```python
from build123d import *

# Parameters (mm, degrees)
F0_W     = 15
F0_H     = 90
F0_R     = 1.5
F1_DEPTH = 3
F2_W     = 15
F2_H     = 3
F3_DEPTH = 17
F4_R     = 2.5
F5_DEPTH = 53.001


with BuildPart() as f1:
    # F0 (on Front) → F1 (new body)
    with BuildSketch(Plane.XZ):
        Rectangle(F0_W, F0_H)
        with Locations((0, -41)):
            Circle(F0_R, mode=Mode.SUBTRACT)
        with Locations((0, 41)):
            Circle(F0_R, mode=Mode.SUBTRACT)
    extrude(amount=F1_DEPTH)

    # F2 (on face) → F3 (join)
    with BuildSketch(Plane.XZ.offset(3)):
        with Locations((0, 6.5)):
            Rectangle(F2_W, F2_H)
    extrude(amount=F3_DEPTH)

    # F4 (on face) → F5 (cut, through all)
    with BuildSketch(Plane.XY.offset(8)):
        with Locations((0, -11.5)):
            Circle(F4_R)
    extrude(amount=-F5_DEPTH, mode=Mode.SUBTRACT)


solid = f1.part
```
The model under review builds one solid part; all positions refer to its coordinate system, in mm. A direction names the side the tool comes from. Coordinates: 2 decimals unless noted, no trailing zeros. Write each loop counter-clockwise with the first axis right and the second up, starting at its lowest first coordinate (ties: lowest second). Pieces come first, ordered by that corner, then holes.
1) The part is to be moulded in two halves that separate along X. For faces 4 (the face through (0, -3, -20)), 5 (the face through (7.5, -2.5, -0.2)), 6 (the face through (-0.325, -1.479, 39.536)), say which applies: pulls with the +X half, pulls with the -X half, needs draft (parallel to the pull), parting line crosses it, or undercut.
2) We need section C-C on x = 0. State the section outline as (y, z) points.
3) We need section A-A on z = 41. State the section outline as (x, y) points.
4) We need section D-D on x = 6. State the section outline as (y, z) points, then the cut area to 3 significant figures.
5) Clearance check with flat-ended pins moving along their axes: pin 1 Ø12 at (y, z) = (-7, 15.5) entering from +X; pin 2 Ø6 at (x, y) = (0, -11.5) entering from -Z; pin 3 Ø7.5 at (x, z) = (-3.5, 20.5) entering from -Y; pin 4 Ø2 at (x, y) = (0.5, -15.5) entering from +Z. State where each tip first meets the part, or that it passes through.
6) To check wall thickness, follow probe 1 along Z at (x, y) = (0, -2.4); probe 2 along Z at (x, y) = (-3, -4); probe 3 along Y at (x, z) = (5.75, -26). State the ranges of each line that lie inside material, in increasing order.
7) We need section B-B on y = -13. State the section outline as (x, z) points.
8) Machinability: for faces 1 (the face through (-2, -9, 5)), 2 (the face through (-7.5, -2.5, -0.2)), 3 (the face through (-2, -9, 8)), which of the approach directions +Z, -Z, +X, -X, +Y, -Y give a long, thin tool a straight path to every point of the face, cutting with its end or side? Answer none if there is none.
Answer list:
1. face 4: needs draft
1. face 5: pulls with the +X half
1. face 6: undercut
2. outline: (-20, 5) - (-14, 5) - (-14, 8) - (-20, 8) - close; (-9, 5) - (-3, 5) - (-3, -39.5) - (0, -39.5) - (0, 39.5) - (-3, 39.5) - (-3, 8) - (-9, 8) - close; (-3, -45) - (0, -45) - (0, -42.5) - (-3, -42.5) - close; (-3, 42.5) - (0, 42.5) - (0, 45) - (-3, 45) - close
3. outline: (-7.5, -3) - (-1.5, -3) - (-1.5, 0) - (-7.5, 0) - close; (1.5, -3) - (7.5, -3) - (7.5, 0) - (1.5, 0) - close
4. outline: (-20, 5) - (-3, 5) - (-3, -45) - (0, -45) - (0, 45) - (-3, 45) - (-3, 8) - (-20, 8) - close
4. area: 321 mm2
5. pin 1: stops at x = 7.5
5. pin 2: stops at z = 5
5. pin 3: stops at y = -3
5. pin 4: stops at z = 8
6. probe 1: z = -45 to -42.5, -39.5 to 39.5, 42.5 to 45
6. probe 2: z = 5 to 8
6. probe 3: y = -3 to 0
7. outline: (-7.5, 5) - (-2, 5) - (-2, 8) - (-7.5, 8) - close; (2, 5) - (7.5, 5) - (7.5, 8) - (2, 8) - close
8. face 1: -Z, +X, -X, -Y
8. face 2: +Z, -Z, -X, +Y, -Y
8. face 3: +Z, +X, -X, -Y
